from build123d import *

# Parameters (mm, degrees)
SKIZZE1_W                            = 71.8
SKIZZE1_H                            = 158
AUFSATZ_LINEAR_AUSTRAGEN1_DEPTH      = 10.25
VERRUNDUNG1_R                        = 10
VERRUNDUNG2_R                        = 3
VERRUNDUNG3_R                        = 0.5
SCHNITT_LINEAR_AUSTRAGEN_D_NN1_DEPTH = 0.5
SCHNITT_LINEAR_AUSTRAGEN_D_NN2_DEPTH = 0.5
SKIZZE4_R                            = 2.6
SKIZZE4_R_2                          = 2.5
SCHNITT_LINEAR_AUSTRAGEN_D_NN3_DEPTH = 0.5
AUFSATZ_LINEAR_AUSTRAGEN2_DEPTH      = 0.5
SKIZZE6_R                            = 1.875
SKIZZE6_R_2                          = 0.65
SCHNITT_LINEAR_AUSTRAGEN1_DEPTH      = 25
SKIZZE7_R                            = 0.65
SCHNITT_LINEAR_AUSTRAGEN2_DEPTH      = 7
SKIZZE8_R                            = 5.25
SCHNITT_LINEAR_AUSTRAGEN3_DEPTH      = 0.9
FASE1_SIZE                           = 0.8
SCHNITT_LINEAR_AUSTRAGEN4_DEPTH      = 0.3
FASE2_SIZE                           = 0.2
SKIZZE10_W                           = 64.08
SKIZZE10_H                           = 129.6
SKIZZE10_W_2                         = 63.88
SKIZZE10_H_2                         = 129.4
SCHNITT_LINEAR_AUSTRAGEN_D_NN4_DEPTH = 0.01
SCHNITT_LINEAR_AUSTRAGEN5_DEPTH      = 2


with BuildPart() as part:
    # Skizze1 → Aufsatz-Linear austragen1 (new body)
    with BuildSketch(Plane(origin=(0, 0, 0), x_dir=(1, 0, 0), z_dir=(0, 1, 0))):
        Rectangle(SKIZZE1_W, SKIZZE1_H)
    extrude(amount=AUFSATZ_LINEAR_AUSTRAGEN1_DEPTH)

    # Verrundung1
    verrundung1_edges = [part.edges().sort_by_distance(p)[0] for p in [
        (35.9, 5.125, 79),
        (-35.9, 5.125, 79),
        (-35.9, 5.125, -79),
        (35.9, 5.125, -79),
    ]]
    fillet(verrundung1_edges, radius=VERRUNDUNG1_R)

    # Verrundung2
    verrundung2_edges = [part.edges().sort_by_distance(p)[0] for p in [
        (-35.9, 0, 0),
        (35.9, 0, 0),
        (0, 0, 79),
        (0, 0, -79),
        (32.971067812, 0, 76.071067812),
        (-32.971067812, 0, 76.071067812),
        (32.971067812, 0, -76.071067812),
        (-32.971067812, 0, -76.071067812),
    ]]
    fillet(verrundung2_edges, radius=VERRUNDUNG2_R)

    # Verrundung3
    verrundung3_edges = [part.edges().sort_by_distance(p)[0] for p in [
        (-35.9, 10.25, 0),
        (0, 10.25, -79),
        (35.9, 10.25, 0),
        (0, 10.25, 79),
        (32.971067812, 10.25, 76.071067812),
        (-32.971067812, 10.25, 76.071067812),
        (32.971067812, 10.25, -76.071067812),
        (-32.971067812, 10.25, -76.071067812),
    ]]
    fillet(verrundung3_edges, radius=VERRUNDUNG3_R)

    # Skizze2 → Schnitt-Linear-Austragen-Dünn1 (cut)
    with BuildSketch(Plane(origin=(0, 10.25, 0), x_dir=(1, 0, 0), z_dir=(0, 1, 0))):
        with BuildLine():
            Line((-27.75, 76.575), (27.75, 76.575))
            ThreePointArc((27.75, 76.575), (32.346194078, 74.671194078), (34.25, 70.075))
            Line((34.25, 70.075), (34.25, -70.075))
            ThreePointArc((34.25, -70.075), (32.346194078, -74.671194078), (27.75, -76.575))
            Line((27.75, -76.575), (-27.75, -76.575))
            ThreePointArc((-27.75, -76.575), (-32.346194078, -74.671194078), (-34.25, -70.075))
            Line((-34.25, -70.075), (-34.25, 70.075))
            ThreePointArc((-34.25, 70.075), (-32.346194078, 74.671194078), (-27.75, 76.575))
        make_face()
        with BuildLine():
            Line((-27.75, 76.475), (27.75, 76.475))
            ThreePointArc((27.75, 76.475), (32.2754834, 74.6004834), (34.15, 70.075))
            Line((34.15, 70.075), (34.15, -70.075))
            ThreePointArc((34.15, -70.075), (32.2754834, -74.6004834), (27.75, -76.475))
            Line((27.75, -76.475), (-27.75, -76.475))
            ThreePointArc((-27.75, -76.475), (-32.2754834, -74.6004834), (-34.15, -70.075))
            Line((-34.15, -70.075), (-34.15, 70.075))
            ThreePointArc((-34.15, 70.075), (-32.2754834, 74.6004834), (-27.75, 76.475))
        make_face(mode=Mode.SUBTRACT)
    extrude(amount=-SCHNITT_LINEAR_AUSTRAGEN_D_NN1_DEPTH, mode=Mode.SUBTRACT)

    # Skizze3 → Schnitt-Linear-Austragen-Dünn2 (cut)
    with BuildSketch(Plane(origin=(0, 10.25, 0), x_dir=(1, 0, 0), z_dir=(0, 1, 0))):
        with BuildLine():
            Line((-0.01, 71.475), (0.01, 71.475))
            ThreePointArc((0.01, 71.475), (1.770695885, 72.204304115), (2.5, 73.965))
            Line((2.5, 73.965), (2.5, 76.475))
            Line((2.5, 76.475), (-2.5, 76.475))
            Line((-2.5, 76.475), (-2.5, 73.965))
            ThreePointArc((-2.5, 73.965), (-1.770695885, 72.204304115), (-0.01, 71.475))
        make_face()
        with BuildLine():
            Line((-0.01, 71.575), (0.01, 71.575))
            ThreePointArc((0.01, 71.575), (1.699985207, 72.275014793), (2.4, 73.965))
            Line((2.4, 73.965), (2.4, 76.375))
            Line((2.4, 76.375), (-2.4, 76.375))
            Line((-2.4, 76.375), (-2.4, 73.965))
            ThreePointArc((-2.4, 73.965), (-1.699985207, 72.275014793), (-0.01, 71.575))
        make_face(mode=Mode.SUBTRACT)
    extrude(amount=-SCHNITT_LINEAR_AUSTRAGEN_D_NN2_DEPTH, mode=Mode.SUBTRACT)

    # Skizze4 → Schnitt-Linear-Austragen-Dünn3 (cut)
    with BuildSketch(Plane(origin=(0, 10.25, 0), x_dir=(1, 0, 0), z_dir=(0, 1, 0))):
        with Locations((6.5, 71.575)):
            Circle(SKIZZE4_R)
        with Locations((6.5, 71.575)):
            Circle(SKIZZE4_R_2, mode=Mode.SUBTRACT)
    extrude(amount=-SCHNITT_LINEAR_AUSTRAGEN_D_NN3_DEPTH, mode=Mode.SUBTRACT)

    # Skizze5 → Aufsatz-Linear austragen2 (add)
    with BuildSketch(Plane.ZY.offset(35.9)):
        with BuildLine():
            Line((-45.7, 4.61), (-36.1, 4.61))
            Line((-36.1, 4.61), (-36.1, 7.25))
            Line((-36.1, 7.25), (-45.7, 7.25))
            ThreePointArc((-45.7, 7.25), (-46.619238816, 6.869238816), (-47, 5.95))
            Line((-47, 5.95), (-47, 5.91))
            ThreePointArc((-47, 5.91), (-46.619238816, 4.990761184), (-45.7, 4.61))
        make_face()
        with BuildLine():
            Line((-24.2, 7.25), (-33.8, 7.25))
            Line((-33.8, 7.25), (-33.8, 4.61))
            Line((-33.8, 4.61), (-24.2, 4.61))
            ThreePointArc((-24.2, 4.61), (-23.280761184, 4.990761184), (-22.9, 5.91))
            Line((-22.9, 5.91), (-22.9, 5.95))
            ThreePointArc((-22.9, 5.95), (-23.280761184, 6.869238816), (-24.2, 7.25))
        make_face()
        with BuildLine():
            Line((-5.5, 7.25), (-13.95, 7.25))
            ThreePointArc((-13.95, 7.25), (-14.869238816, 6.869238816), (-15.25, 5.95))
            Line((-15.25, 5.95), (-15.25, 5.91))
            ThreePointArc((-15.25, 5.91), (-14.869238816, 4.990761184), (-13.95, 4.61))
            Line((-13.95, 4.61), (-5.5, 4.61))
            ThreePointArc((-5.5, 4.61), (-4.580761184, 4.990761184), (-4.2, 5.91))
            Line((-4.2, 5.91), (-4.2, 5.95))
            ThreePointArc((-4.2, 5.95), (-4.580761184, 6.869238816), (-5.5, 7.25))
        make_face()
    extrude(amount=AUFSATZ_LINEAR_AUSTRAGEN2_DEPTH)

    # Skizze6 → Schnitt-Linear austragen1 (cut)
    with BuildSketch(Plane(origin=(0, 0, -79), x_dir=(-1, 0, 0), z_dir=(0, 0, -1))):
        with Locations((23.4, 4.55)):
            Circle(SKIZZE6_R)
        with Locations((12.4, 6)):
            Circle(SKIZZE6_R_2)
    extrude(amount=-SCHNITT_LINEAR_AUSTRAGEN1_DEPTH, mode=Mode.SUBTRACT)

    # Skizze7 → Schnitt-Linear austragen2 (cut)
    with BuildSketch(Plane.XY.offset(79)):
        with Locations((6.4, 5.8)):
            Circle(SKIZZE7_R)
        with BuildLine():
            Line((-8.2, 6.75), (-2.5, 6.75))
            ThreePointArc((-2.5, 6.75), (-1, 5.25), (-2.5, 3.75))
            Line((-2.5, 3.75), (-8.2, 3.75))
            ThreePointArc((-8.2, 3.75), (-9.7, 5.25), (-8.2, 6.75))
        make_face()
    extrude(amount=-SCHNITT_LINEAR_AUSTRAGEN2_DEPTH, mode=Mode.SUBTRACT)

    # Skizze8 → Schnitt-Linear austragen3 (cut)
    with BuildSketch(Plane.XZ):
        with Locations(Location((0, -55.5, 0), (0, 0, 270))):
            Circle(SKIZZE8_R)
    extrude(amount=-SCHNITT_LINEAR_AUSTRAGEN3_DEPTH, mode=Mode.SUBTRACT)

    # Fase1
    fase1_edges = [part.edges().sort_by_distance(p)[0] for p in [
        (0, 0, -50.25),
    ]]
    chamfer(fase1_edges, length=FASE1_SIZE)

    # Skizze9 → Schnitt-Linear austragen4 (cut)
    with BuildSketch(Plane.XZ):
        with BuildLine():
            Line((25.4, -74.5), (16.5, -74.5))
            ThreePointArc((16.5, -74.5), (11, -69), (16.5, -63.5))
            Line((16.5, -63.5), (25.4, -63.5))
            ThreePointArc((25.4, -63.5), (30.9, -69), (25.4, -74.5))
        make_face()
    extrude(amount=-SCHNITT_LINEAR_AUSTRAGEN4_DEPTH, mode=Mode.SUBTRACT)

    # Fase2
    fase2_edges = [part.edges().sort_by_distance(p)[0] for p in [
        (30.9, 0, -69),
        (20.95, 0, -63.5),
        (11, 0, -69),
        (20.95, 0, -74.5),
    ]]
    chamfer(fase2_edges, length=FASE2_SIZE)

    # Skizze10 → Schnitt-Linear-Austragen-Dünn4 (cut)
    with BuildSketch(Plane(origin=(0, 10.25, 0), x_dir=(1, 0, 0), z_dir=(0, 1, 0))):
        Rectangle(SKIZZE10_W, SKIZZE10_H)
        Rectangle(SKIZZE10_W_2, SKIZZE10_H_2, mode=Mode.SUBTRACT)
    extrude(amount=-SCHNITT_LINEAR_AUSTRAGEN_D_NN4_DEPTH, mode=Mode.SUBTRACT)

    # Skizze11 → Schnitt-Linear austragen5 (cut)
    with BuildSketch(Plane.ZY.offset(35.9)):
        with BuildLine():
            Line((56.1, 6.25), (60.9, 6.25))
            ThreePointArc((60.9, 6.25), (61.8, 5.35), (60.9, 4.45))
            Line((60.9, 4.45), (56.1, 4.45))
            ThreePointArc((56.1, 4.45), (55.2, 5.35), (56.1, 6.25))
        make_face()
        with BuildLine():
            Line((63.55, 6.25), (68.35, 6.25))
            ThreePointArc((68.35, 6.25), (69.25, 5.35), (68.35, 4.45))
            Line((68.35, 4.45), (63.55, 4.45))
            ThreePointArc((63.55, 4.45), (62.65, 5.35), (63.55, 6.25))
        make_face()
        with BuildLine():
            Line((41.55, 4.3), (48.9, 4.3))
            ThreePointArc((48.9, 4.3), (49.819238816, 3.919238816), (50.2, 3))
            Line((50.2, 3), (49.680384758, 2.7))
            Line((49.680384758, 2.7), (40.769615242, 2.7))
            Line((40.769615242, 2.7), (40.25, 3))
            ThreePointArc((40.25, 3), (40.630761184, 3.919238816), (41.55, 4.3))
        make_face()
    extrude(amount=-SCHNITT_LINEAR_AUSTRAGEN5_DEPTH, mode=Mode.SUBTRACT)


solid = part.part
Could you check a few things on this model? Use its own coordinates, in mm. A direction names the side the tool comes from. Coordinates: 2 decimals unless noted, no trailing zeros. Write item = value, one per line.
1) Suppose I cut it at B-B on z = -67. State how many separate pieces and enclosed holes the cut face has, plus the area to 3 significant figures.
Result set:
separate_pieces = 1
enclosed_holes = 2
area = 714 mm2
2) For faces 1 (the cylindrical face through (-25.13, 3.83, -66.68)), 2 (the flat face through (6, 10.25, -72)), 3 (the flat face through (-5, 5, 72)), which set-ups out of +Z, -Z, +X, -X, +Y, -Y let a thin tool reach every point of the face, with its end or its side?
Result set:
face_1 = -Z
face_2 = +Z, -Z, +X, -X, +Y
face_3 = +Z
3) Please list where these lines run through material, in increasing order: line 1 (Y direction, x = -12.4, z = -61); line 2 (Y direction, x = 6.4, z = 73.75); line 3 (X direction, y = 4.55, z = -62) (3 decimals). Write a range as [from, to].
Result set:
line_1 = [0, 5.35], [6.65, 10.25]
line_2 = [0, 5.15], [6.45, 10.25]
line_3 = [-35.9, -25.275], [-21.525, 35.9]
4) Will these pins go through, and if not, where does the flat tip stop? pin 1 Ø1.5 at (y, z) = (9, -30.5) entering from -X; pin 2 Ø0.8 at (y, z) = (3.5, 45.5) entering from -X.
Result set:
pin_1 = -35.9
pin_2 = -33.9
